Can you work these out from the model? Positions are in its coordinate system, mm. A direction names the side the tool comes from. Round coordinates to 2 decimals unless told otherwise and drop trailing zeros. Order: outer loops, then holes, each group sorted by start corner. A loop starts at its lowest first (then second) coordinate and runs counter-clockwise, first axis right, second up. Notation, with made-up numbers: M 0,-27.5 L 51,-27.5 A21 cw 51,-14.5 Z; hole C -8.75,36 d3. An arc over 180 degrees is marked long. One line per question, with ' | ' between items.
```python
from build123d import *

# Parameters (mm, degrees)
ESBO_O1_W                = 6
ESBO_O1_H                = 5
RESSALTO_EXTRUS_O1_DEPTH = 5
ESBO_O3_W                = 2.2
ESBO_O3_H                = 4
CORTE_EXTRUS_O1_DEPTH    = 5
FILETE1_R                = 1
FILETE2_R                = 1
FILETE3_R                = 1
FILETE4_R                = 1
FILETE5_R                = 0.5
FILETE6_R                = 0.5
FILETE7_R                = 0.3
FILETE8_R                = 0.3


with BuildPart() as part:
    # Esboço1 → Ressalto-extrusão1 (new body)
    with BuildSketch(Plane(origin=(0, 0, 0), x_dir=(1, 0, 0), z_dir=(0, 1, 0))):
        Rectangle(ESBO_O1_W, ESBO_O1_H)
    extrude(amount=RESSALTO_EXTRUS_O1_DEPTH)

    # Esboço3 → Corte-extrusão1 (cut)
    with BuildSketch(Plane(origin=(0, 5, 0), x_dir=(1, 0, 0), z_dir=(0, 1, 0))):
        with Locations((0.4, 0.5)):
            Rectangle(ESBO_O3_W, ESBO_O3_H)
    extrude(amount=-CORTE_EXTRUS_O1_DEPTH, mode=Mode.SUBTRACT)

    # Filete1
    filete1_edges = [part.edges().sort_by_distance(p)[0] for p in [
        (3, 2.5, 2.5),
    ]]
    fillet(filete1_edges, radius=FILETE1_R)

    # Filete2
    filete2_edges = [part.edges().sort_by_distance(p)[0] for p in [
        (-3, 2.5, 2.5),
    ]]
    fillet(filete2_edges, radius=FILETE2_R)

    # Filete3
    filete3_edges = [part.edges().sort_by_distance(p)[0] for p in [
        (-3, 2.5, -2.5),
    ]]
    fillet(filete3_edges, radius=FILETE3_R)

    # Filete4
    filete4_edges = [part.edges().sort_by_distance(p)[0] for p in [
        (-0.7, 2.5, -2.5),
    ]]
    fillet(filete4_edges, radius=FILETE4_R)

    # Filete5
    filete5_edges = [part.edges().sort_by_distance(p)[0] for p in [
        (1.5, 2.5, -2.5),
    ]]
    fillet(filete5_edges, radius=FILETE5_R)

    # Filete6
    filete6_edges = [part.edges().sort_by_distance(p)[0] for p in [
        (3, 2.5, -2.5),
    ]]
    fillet(filete6_edges, radius=FILETE6_R)

    # Filete7
    filete7_edges = [part.edges().sort_by_distance(p)[0] for p in [
        (1.5, 2.5, 1.5),
    ]]
    fillet(filete7_edges, radius=FILETE7_R)

    # Filete8
    filete8_edges = [part.edges().sort_by_distance(p)[0] for p in [
        (-0.7, 2.5, 1.5),
    ]]
    fillet(filete8_edges, radius=FILETE8_R)


solid = part.part
```
(1) If we section it at A-A on z = 1.1: Please give me the cut outline in (x, y), plus the area to 3 significant figures.
Final values:
outline: M -3,0 L -0.7,0 L -0.7,5 L -3,5 Z; M 1.5,0 L 3,0 L 3,5 L 1.5,5 Z | area: 19.0 mm^2
(2) If we section it at B-B on y = 0.45: Please give me the cut outline in (x, z), plus the area to 3 significant figures.
Final values:
outline: M -3,-1.5 A1 ccw -2,-2.5 L -1.7,-2.5 A1 ccw -0.7,-1.5 L -0.7,1.2 A0.3 cw -0.4,1.5 L 1.2,1.5 A0.3 cw 1.5,1.2 L 1.5,-2 A0.5 ccw 2,-2.5 L 2.5,-2.5 A0.5 ccw 3,-2 L 3,1.5 A1 ccw 2,2.5 L -2,2.5 A1 ccw -3,1.5 Z | area: 20.3 mm^2
(3) If we section it at C-C on x = 0.9: Please give me the cut outline in (y, z).
Final values:
outline: M 0,1.5 L 5,1.5 L 5,2.5 L 0,2.5 Z
(4) Please list where these lines run through material, in increasing order: probe 1 along X at (y, z) = (1.75, 0.6); probe 2 along Z at (x, y) = (-0.2, 4.1); probe 3 along X at (y, z) = (3.05, 1.4). Write a range as [from, to].
Final values:
probe 1: [-3, -0.7], [1.5, 3] | probe 2: [1.5, 2.5] | probe 3: [-3, -0.62], [1.42, 3]
(5) Will these pins go through, and if not, where does the flat tip stop? pin 1 Ø1 at (x, y) = (0, 3) entering from -Z; pin 2 Ø1.5 at (x, z) = (1, -1) entering from -Y.
Final values:
pin 1: z = 1.48 | pin 2: y = 0
(6) Thinking about a two-plate mould opening in X: for faces 3 (the cylindrical face through (-2.699, 2.535, 2.215)), 4 (the flat face through (3, 2, 0)), 5 (the cylindrical face through (-1.001, 2.465, -2.215)), 6 (the flat face through (0, 3, 1.5)), which applies, released by +X, released by -X, zero draft, split by the parting line, or undercut?
Final values:
face 3: released by -X | face 4: released by +X | face 5: undercut | face 6: undercut
(7) If we section it at D-D on z = 2.05: Please give me the cut outline in (x, y).
Final values:
outline: M -2.84,0 L 2.84,0 L 2.84,5 L -2.84,5 Z
(8) On a 3-axis mill with a long thin cutter (end or side, diameter ignored), from which of +Z, -Z, +X, -X, +Y, -Y can I reach the whole of each face in a straight line? I mean faces 1 (the flat face through (-0.7, 3, 0)), 2 (the flat face through (-1, 5, 1)). Say none if no direction works.
Final values:
face 1: -Z, +Y, -Y | face 2: +Z, -Z, +X, -X, +Y
